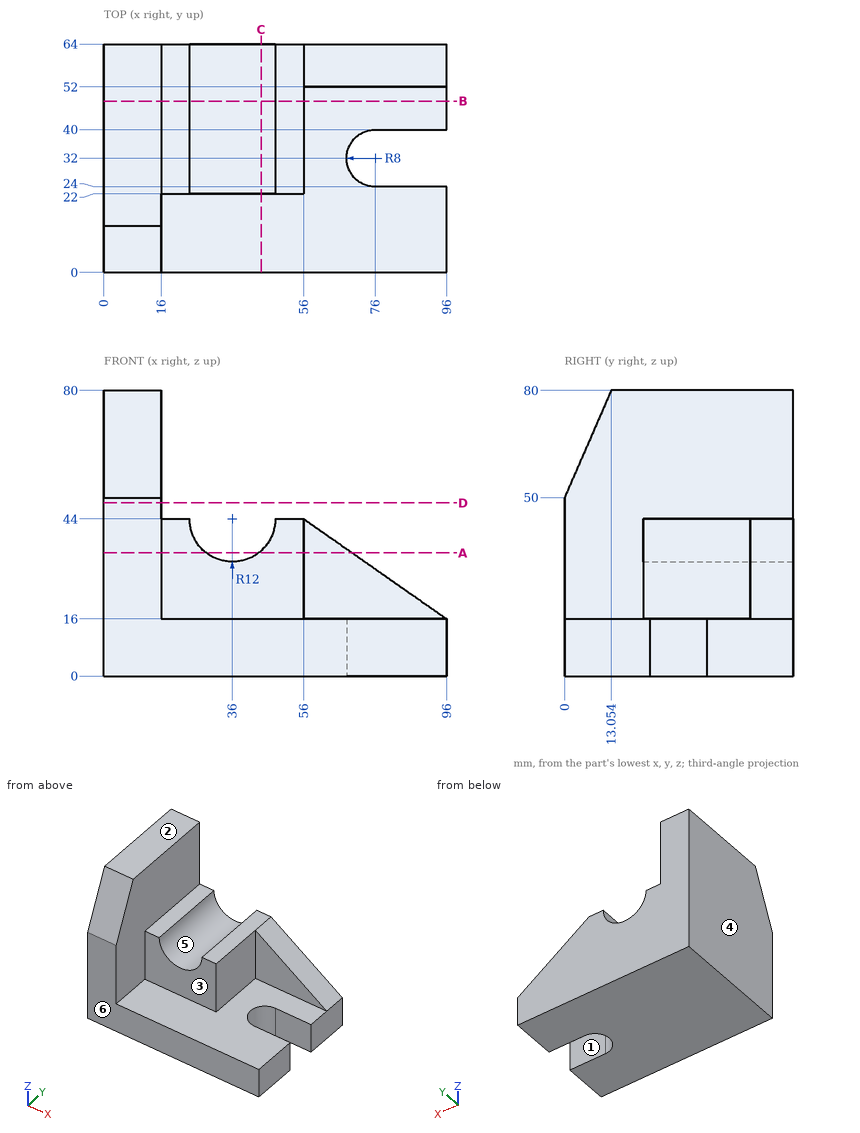
Job drawing, mm, ordinate dimensions from the low corner. One solid piece. A direction names the side the tool comes from. Coordinates: 2 decimals unless noted, no trailing zeros. Order: outer loops, then holes, each group sorted by start corner. A loop starts at its lowest first (then second) coordinate and runs counter-clockwise, first axis right, second up. Notation, with made-up numbers: (34, 40.5) -> (43, 40.5) arc R20 cw to (43, 79.5) -> close; hole circle Ø2 at (51.25, 76.5). An arc over 180 degrees is marked (long way). Put each result on its own line as item: value. Start each with the question number.
(1) Band-saw the part on C-C (x = 44). Give the cut face in (y, z), then the cut area to 3 significant figures.
(2) Band-saw the part on A-A (z = 34.5). Give the cut face in (x, y).
(3) Probe line 1 along Y through (x, z) = (77.5, 10); line 2 along X through (y, z) = (37, 43.5); line 3 along X through (y, z) = (4, 23.5). List the from-to ranges inside material, lowest first. Write a range as [from, to].
(4) Which spindle directions (+Z, -Z, +X, -X, +Y, -Y) get a long thin tool onto all of the face, cutting with end or side? Do the marked faces 1, 2 and 3. Say none if no direction does.
(5) Band-saw the part on D-D (z = 48.5). Give the cut face in (x, y), then the cut area to 3 significant figures.
(6) Pin check, flat tips, straight feed: pin 1 Ø8.5 at (x, z) = (67, 34) entering from -Y; pin 2 Ø8 at (x, y) = (20.5, 30) entering from +Z; pin 3 Ø6 at (x, y) = (83, 44.5) entering from +Z. Stop position of each tip, or through.
(7) Mould opens along X. For the marked faces 4, 5 and 6 say: pulls with the +X half, pulls with the -X half, needs draft (parallel to the pull), parting line crosses it, or undercut.
(8) Band-saw the part on B-B (y = 48). Give the cut face in (x, z), then the cut area to 3 significant figures.
Determined:
1. outline: (0, 0) -> (64, 0) -> (64, 35.06) -> (22, 35.06) -> (22, 16) -> (0, 16) -> close
1. area: 1,820 mm²
2. outline: (0, 0) -> (16, 0) -> (16, 22) -> (28.67, 22) -> (28.67, 64) -> (0, 64) -> close; (43.33, 22) -> (56, 22) -> (56, 52) -> (69.57, 52) -> (69.57, 64) -> (43.33, 64) -> close
3. line 1: y = [0, 24], [40, 64]
3. line 2: x = [0, 24.01], [47.99, 56]
3. line 3: x = [0, 16]
4. face 1: +Z, -Z, +X
4. face 2: +Z, +X, -X, +Y, -Y
4. face 3: +Z, +X, -Y
5. outline: (0, 0) -> (16, 0) -> (16, 64) -> (0, 64) -> close
5. area: 1,020 mm²
6. pin 1: stops at y = 52
6. pin 2: stops at z = 44
6. pin 3: stops at z = 16
7. face 4: pulls with the -X half
7. face 5: undercut
7. face 6: needs draft
8. outline: (0, 0) -> (96, 0) -> (96, 16) -> (56, 16) -> (56, 44) -> (48, 44) arc R12 cw to (24, 44) -> (16, 44) -> (16, 80) -> (0, 80) -> close
8. area: 3,450 mm²
